Build history of the part. All positions in model axes, mm. A direction names the side the tool comes from. Coordinates: 2 decimals unless noted, no trailing zeros. Write each loop counter-clockwise with the first axis right and the second up, starting at its lowest first coordinate (ties: lowest second). Pieces come first, ordered by that corner, then holes.
Solid Edge part; units mm, degrees
sketch "Sketch1" plane through (0, 0, 0) normal (0, 0, 1) x (1, 0, 0)
  line L0 (-3, -3) -> (3, -3)
  line L1 (3, -3) -> (3, 3)
  line L2 (3, 3) -> (-3, 3)
  line L3 (-3, 3) -> (-3, -3)
extrude "Protrusion1" add sketch "Sketch1" against normal blind 3.4
sketch "Sketch2" plane through (0, 0, 0) normal (0, 0, 1) x (1, 0, 0)
  circle A0 centre (0, 0) radius 1.75
extrude "ExtrudedProtrusion_2" add sketch "Sketch2" along normal blind 1.6
sketch "Sketch3" plane through (0, 0, 0) normal (0, 0, 1) x (1, 0, 0)
  circle A0 centre (-2.2, -2.1954) radius 0.5
extrude "ExtrudedProtrusion_3" add sketch "Sketch3" along normal blind 0.5
pattern_circular "Pattern1" count 4 over 360 about axis through (0, 0, 0) along (0, 0, -1) of "ExtrudedProtrusion_3"
extrude "ExtrudedProtrusion_4" [suppressed]
sketch "Sketch4" plane through (0, 3, -1.7) normal (0, 1, 0) x (0, 0, -1)
  line L0 (0.7, -1.9) -> (1.3987, -1.9)
  line L1 (1.3987, -1.9) -> (1.3987, -2.6)
  line L2 (1.3987, -2.6) -> (0.7, -2.6)
  line L3 (0.7, -2.6) -> (0.7, -1.9)
  line L4 (0.7, 2.6) -> (1.3987, 2.6)
  line L5 (1.3987, 2.6) -> (1.3987, 1.9)
  line L6 (1.3987, 1.9) -> (0.7, 1.9)
  line L7 (0.7, 1.9) -> (0.7, 2.6)
extrude "ExtrudedProtrusion_5" add sketch "Sketch4" along normal blind 4
(1) Probe L1, parallel to X at y = 6, z = -3; L2, parallel to Z at x = -0.8, y = -2; L3, parallel to Y at x = 1.35, z = -2.1. List the from-to ranges inside material, lowest first.
(2) Slice it at B-B, the plane x = 0. List the corners of the cut face in (y, z).
(3) Slice it at A-A, the plane y = 6.25. List the corners of the cut face in (x, z), and give its area (3 significant figures).
(4) Flat gauge pins, fed straight in: P1, Ø1, axis at x = 2, y = 1.5, coming from the +Z side; P2, Ø2, axis at x = -1, y = 5, coming from the -Z side; P3, Ø0.6, axis at y = 4.5, z = -3, coming from the +X side. Where does each tip first touch, or does it go through?
(5) Slice it at D-D, the plane z = -0.5. List the corners of the cut face in (x, y), and give its area (3 significant figures).
(6) 3-axis set-ups, long thin cutter, end or side, ignore diameter. For faces 5 (the cylindrical face through (1.617, 0.67, 0.789)), 6 (the flat face through (0, 0, -3.4)): which of +Z, -Z, +X, -X, +Y, -Y reach the whole face in a straight line?
(7) Two-plate mould, pull along X, no slides. Class faces 1 (the flat face through (0, 0, 1.6)), 2 (the flat face through (-3, 0, -2)), 3 (the cylindrical face through (2.69, -2.27, 0.25)), 4 (the flat face through (3, 0, -2)): pulls with the +X half, pulls with the -X half, needs draft (parallel to the pull), parting line crosses it, or undercut.
Results:
1. L1: x = -2.6 to -1.9, 1.9 to 2.6
1. L2: z = -3.4 to 0
1. L3: y = -3 to 3
2. outline: (-3, -3.4) - (3, -3.4) - (3, 0) - (1.75, 0) - (1.75, 1.6) - (-1.75, 1.6) - (-1.75, 0) - (-3, 0) - close
3. outline: (-2.6, -3.1) - (-1.9, -3.1) - (-1.9, -2.4) - (-2.6, -2.4) - close; (1.9, -3.1) - (2.6, -3.1) - (2.6, -2.4) - (1.9, -2.4) - close
3. area: 0.978 mm2
4. P1: stops at z = 0.5
4. P2: stops at z = -3.1
4. P3: stops at x = 2.6
5. outline: (-3, -3) - (3, -3) - (3, 3) - (-3, 3) - close
5. area: 36.0 mm2
6. face 5: +Z
6. face 6: -Z, +X, -X, +Y, -Y
7. face 1: needs draft
7. face 2: pulls with the -X half
7. face 3: undercut
7. face 4: pulls with the +X half
